Autodesk Inventor part; units mm, degrees
ref_plane "YZ Plane" through (0, 0, 0) normal (1, 0, 0) x (0, 1, 0)
ref_plane "XZ Plane" through (0, 0, 0) normal (0, 1, 0) x (-1, 0, 0)
ref_plane "XY Plane" through (0, 0, 0) normal (0, 0, 1) x (1, 0, 0)
sketch "Sketch1" plane through (0, 0, 0) normal (0, 1, 0) x (-1, 0, 0)
  circle A0 centre (0, 0) radius 12.5
  circle A1 centre (0, 0) radius 16.6
  circle A2 centre (0, 0) radius 18
  circle A3 centre (0, 0) radius 14.75
  dimension "d0" = 25
  dimension "d1" = 33.2
  dimension "d2" = 36
  dimension "d3" = 29.5
extrude "Extrusion1" add sketch "Sketch1" along normal blind 3 contours A1 | A3
sketch "Sketch2" plane through (0, 0, 0) normal (0, -1, 0) x (1, 0, 0)
  circle A0 centre (0, 0) radius 12.5
  circle A1 centre (0, 0) radius 12.5
  circle A2 centre (0, 0) radius 16.6
  circle A3 centre (0, 0) radius 18
  circle A4 centre (0, 0) radius 14.75
  dimension "d6" = 25
  dimension "d7" = 33.2
  dimension "d8" = 36
  dimension "d9" = 29.5
extrude "Extrusion2" add sketch "Sketch2" against normal blind 6.4 contours A0
fillet "Fillet1" radius 1.5 1 edges at (-12.5, 6.4, 0)
fillet "Fillet2" radius 2.95 1 edges at (16.6, 3, 0)
sketch "Sketch5" plane through (0, 0, 0) normal (0, -1, 0) x (1, 0, 0)
  circle A0 centre (0, 0) radius 16.6
  circle A1 centre (0, 0) radius 14.75
  dimension "d23" = 29.5
extrude "Extrusion5" add sketch "Sketch5" along normal blind 17 contours A1
sketch "Sketch7" plane through (0, -17, 0) normal (0, -1, 0) x (1, 0, 0)
  line L0 (4.9559, 9.4025) -> (-5.0441, 9.4025)
  line L1 (-5.0441, 9.4025) -> (-5.0441, -10.5975)
  line L2 (-5.0441, -10.5975) -> (4.9559, -10.5975)
  line L3 (4.9559, -10.5975) -> (4.9559, 9.4025)
  point P0 (0, 0)
  dimension "d30" = 10
  dimension "d32" = 20
extrude "Extrusion7" add sketch "Sketch7" along normal blind 8
sketch "Sketch8" plane through (0, -25, 0) normal (0, -1, 0) x (1, 0, 0)
  line L0 (-1.0467, 9.4141) -> (2.9533, 9.4141)
  line L1 (2.9533, 9.4141) -> (2.9533, -10.5859)
  line L2 (2.9533, -10.5859) -> (-1.0467, -10.5859)
  line L3 (-1.0467, -10.5859) -> (-1.0467, 9.4141)
  point P0 (0, 0)
  dimension "d35" = 4
  dimension "d37" = 20
extrude "Extrusion8" add sketch "Sketch8" along normal blind 3
thread "Thread1"
sketch "Sketch10" plane through (0, -28, 0) normal (0, -1, 0) x (1, 0, 0)
  line L0 (0.0695, 9.4148) -> (2.0695, 9.4148)
  line L1 (2.0695, 9.4148) -> (2.0695, -10.5852)
  line L2 (2.0695, -10.5852) -> (0.0695, -10.5852)
  line L3 (0.0695, -10.5852) -> (0.0695, 9.4148)
  point P0 (0, 0)
  dimension "d46" = 20
  dimension "d48" = 2
extrude "Extrusion10" add sketch "Sketch10" along normal blind 7.5
properties part number "OBSN-30-B" material "Nylon 6"
Geometry: final body of the model. Coordinates: model frame, mm. A direction names the side the tool comes from. Give positions to 0.01 mm unless a question says otherwise; leave off trailing zeros. Write each loop counter-clockwise with the first axis right and the second up, starting at its lowest first coordinate (ties: lowest second). Pieces come first, ordered by that corner, then holes. Notation, with made-up numbers: (87.5, 72) - (114.5, 72) arc R13 cw to (114.5, 76) - close; hole circle Ø2 at (80, -1.5). An arc over 180 degrees is marked (long way). Return JSON: item names as keys, results as strings. Group by question number.
1) Line query: line 1 (Y direction, x = 3.5, z = 7); line 2 (Y direction, x = 5, z = -5.5); line 3 (Z direction, x = -0.5, y = -27). Output: solid intervals per line, ascending.
2) First-contact query: P1, Ø4, axis at x = -2, y = -21.5, coming from the +Z side; P2, Ø1.6, axis at x = 1.5, y = -32.5, coming from the -Z side; P3, Ø1.5, axis at y = -26, z = -1.5, coming from the -X side. Flat tips, straight axial feed; report the tip coordinate or a pass-through.
3) Section A-A on z = 0. Return the cut outline in (x, y).
4) Section B-B on y = -1. Return the cut outline in (x, z).
5) Set-up query: faces 1 (the flat face through (0, -21, -10.598)), 2 (the flat face through (0.07, -32, -1)), 3 (the cylindrical face through (11.923, 3.937, 3.755)), 4 (the flat face through (2.07, -32, 0)). Return all of +Z, -Z, +X, -X, +Y, -Y with unobstructed straight access to the full face (end or side cutting, diameter ignored); none if empty.
6) Section C-C on y = -18.5. Return the cut outline in (x, z).
Filled in:
{
 "1": {"line 1": "y = -25 to 6.4", "line 2": "y = -17 to 6.4", "line 3": "z = -10.59 to 9.41"},
 "2": {"P1": "stops at z = 9.4", "P2": "stops at z = -10.59", "P3": "stops at x = -1.05"},
 "3": {"outline": "(-16.6, 0) - (-14.75, 0) - (-14.75, -17) - (-5.04, -17) - (-5.04, -25) - (-1.05, -25) - (-1.05, -28) - (0.07, -28) - (0.07, -35.5) - (2.07, -35.5) - (2.07, -28) - (2.95, -28) - (2.95, -25) - (4.96, -25) - (4.96, -17) - (14.75, -17) - (14.75, 0) - (16.6, 0) - (16.6, 0.05) arc R2.95 ccw to (13.65, 3) - (12.5, 3) - (12.5, 4.9) arc R1.5 ccw to (11, 6.4) - (-11, 6.4) arc R1.5 ccw to (-12.5, 4.9) - (-12.5, 3) - (-13.65, 3) arc R2.95 ccw to (-16.6, 0.05) - close"},
 "4": {"outline": "circle Ø29.5 at (0, 0)"},
 "5": {"face 1": "-Z, +X, -X, -Y", "face 2": "+Z, -Z, -X, -Y", "face 3": "+Y", "face 4": "+Z, -Z, +X, -Y"},
 "6": {"outline": "(-5.04, -10.6) - (4.96, -10.6) - (4.96, 9.4) - (-5.04, 9.4) - close"}
}
